from build123d import *

# Parameters (mm, degrees)
PAD_DEPTH         = 10
SKETCH001_W       = 10
SKETCH001_H       = 4
SKETCH001_W_2     = 3
POCKET_DEPTH      = 18.580627
POCKET_DEPTH_BACK = -1.421373
SKETCH002_R       = 1.6
POCKET001_DEPTH   = 6.001
SKETCH003_R       = 3.1
POCKET002_DEPTH   = 3
SKETCH004_W       = 2.736464
SKETCH004_H       = 4
POCKET003_DEPTH   = 5


with BuildPart() as part:
    # Sketch → Pad (new body, symmetric)
    with BuildSketch(Plane.XZ):
        with BuildLine():
            ThreePointArc((-8.737986, 10), (-9.998746, 4.978781), (-8.579627, 0))
            Line((-8.579627, 0), (-8.579627, -6))
            Line((-8.579627, -6), (8.579627, -6))
            Line((8.579627, -6), (8.579627, 0))
            ThreePointArc((8.579627, 0), (9.998746, 4.978781), (8.737986, 10))
            Line((5.843163, 6.5), (8.737986, 10))
            ThreePointArc((3.1, 0), (5.527888, 2.804212), (5.843163, 6.5))
            Line((-3.1, 0), (3.1, 0))
            ThreePointArc((-5.843163, 6.5), (-5.527888, 2.804212), (-3.1, 0))
            Line((-5.843163, 6.5), (-8.737986, 10))
        make_face()
    extrude(amount=PAD_DEPTH, both=True)

    # Sketch001 (on Face5 of Pad) → Pocket (cut, two sides)
    with BuildSketch(Plane(origin=(8.579627, 0, 0), x_dir=(0, 0, 1), z_dir=(1, 0, 0))) as pocket_sk:
        with Locations((5, 0)):
            Rectangle(SKETCH001_W, SKETCH001_H)
        with Locations((-4.5, 0)):
            Rectangle(SKETCH001_W_2, SKETCH001_H)
    extrude(amount=-POCKET_DEPTH, mode=Mode.SUBTRACT)
    extrude(pocket_sk.sketch, amount=-POCKET_DEPTH_BACK, mode=Mode.SUBTRACT)

    # Sketch002 (on Face12 of Pocket) → Pocket001 (cut, through all)
    with BuildSketch(Plane(origin=(0, 0, 0), x_dir=(-1, 0, 0), z_dir=(0, 0, 1))):
        with Locations((0, 6)):
            Circle(SKETCH002_R)
        with Locations((0, -6)):
            Circle(SKETCH002_R)
    extrude(amount=-POCKET001_DEPTH, mode=Mode.SUBTRACT)

    # Sketch003 (on Face30 of Pocket001) → Pocket002 (cut)
    with BuildSketch(Plane(origin=(0, 0, 0), x_dir=(-1, 0, 0), z_dir=(0, 0, 1))):
        with Locations((0, 6)):
            Circle(SKETCH003_R)
        with Locations((0, -6)):
            Circle(SKETCH003_R)
    extrude(amount=-POCKET002_DEPTH, mode=Mode.SUBTRACT)

    # Sketch004 (on Face13 of Pocket002) → Pocket003 (cut)
    with BuildSketch(Plane(origin=(0, 0, 0), x_dir=(-1, 0, 0), z_dir=(0, 0, 1))):
        with Locations((-7.211395, 0)):
            Rectangle(SKETCH004_W, SKETCH004_H)
        with Locations((7.211395, 0)):
            Rectangle(SKETCH004_W, SKETCH004_H)
    extrude(amount=-POCKET003_DEPTH, mode=Mode.SUBTRACT)


solid = part.part
Can you work these out from the model? Positions are in its coordinate system, mm. A direction names the side the tool comes from. Give positions to 0.01 mm unless a question says otherwise; leave off trailing zeros. Order: outer loops, then holes, each group sorted by start corner. A loop starts at its lowest first (then second) coordinate and runs counter-clockwise, first axis right, second up. Notation, with made-up numbers: M 73.5,67 L 86.5,67 A15 ccw 86.5,85 Z; hole C 69,62.5 d11. An arc over 180 degrees is marked long. One line per question, with ' | ' between items.
Item 1: Please list where these lines run through material, in increasing order: L1, parallel to Y at x = 0, z = -5; L2, parallel to Y at x = 0, z = -1.8; L3, parallel to X at y = 6, z = -0.7.
Answer block:
L1: y = -10 to -7.6, -4.4 to -2, 2 to 4.4, 7.6 to 10 | L2: y = -10 to -9.1, -2.9 to 2.9, 9.1 to 10 | L3: x = -8.58 to -3.1, 3.1 to 8.58
Item 2: I'm going to push flat-ended pins straight in: pin 1 Ø1.8 at (y, z) = (-4, -2.5) entering from -X; pin 2 Ø5 at (x, y) = (-1.5, 5.5) entering from +Z (3 decimals); pin 3 Ø2 at (y, z) = (-3, 7) entering from -X; pin 4 Ø5 at (x, z) = (1, 3.5) entering from +Y. Where does each tip first touch, or does it pass through?
Answer block:
pin 1: stops at x = -8.58 | pin 2: stops at z = 0.665 | pin 3: stops at x = -9.96 | pin 4: passes through
Item 3: For faces 1 (the face through (-5.843, 0, -1)), 2 (the face through (-5.548, -6.056, 2.853)), 3 (the face through (0.672, -2.974, -1.479)), 4 (the face through (-7.27, 5.944, 8.226)), 5 (the face through (8.58, 6, -3)), which set-ups out of +Z, -Z, +X, -X, +Y, -Y let a thin tool reach every point of the face, with its end or its side?
Answer block:
face 1: +Z, -Z, -X | face 2: +Y, -Y | face 3: +Z | face 4: +Z, +Y, -Y | face 5: -Z, +X, +Y, -Y
Item 4: Suppose I cut it at C-C, the plane z = -0.5. Write out the boundary of the cut face in (x, y).
Answer block:
outline: M -8.58,-10 L 8.58,-10 L 8.58,-2 L 5.84,-2 L 5.84,2 L 8.58,2 L 8.58,10 L -8.58,10 L -8.58,2 L -5.84,2 L -5.84,-2 L -8.58,-2 Z; hole C 0,-6 d6.2; hole C 0,6 d6.2
Item 5: Suppose I cut it at D-D, the plane z = 7.75. Write out the boundary of the cut face in (x, y), then the cut area to 3 significant figures.
Answer block:
outline: M -9.65,-10 L -6.88,-10 L -6.88,-2 L -9.65,-2 Z; M -9.65,2 L -6.88,2 L -6.88,10 L -9.65,10 Z; M 6.88,-10 L 9.65,-10 L 9.65,-2 L 6.88,-2 Z; M 6.88,2 L 9.65,2 L 9.65,10 L 6.88,10 Z | area: 88.8 mm2
Item 6: Suppose I cut it at A-A, the plane z = -3.75. Write out the boundary of the cut face in (x, y).
Answer block:
outline: M -8.58,-10 L 8.58,-10 L 8.58,-2 L -8.58,-2 Z; M -8.58,2 L 8.58,2 L 8.58,10 L -8.58,10 Z; hole C 0,-6 d3.2; hole C 0,6 d3.2
Item 7: We'd pull the mould along X, two halves only. Please class faces 6 (the face through (10, 6, 5)), 7 (the face through (-8.58, 6, -3)), 8 (the face through (-5.548, 5.944, 2.853)), 9 (the face through (0, -10, -1)): released by +X, released by -X, zero draft, split by the parting line, or undercut.
Answer block:
face 6: released by +X | face 7: released by -X | face 8: undercut | face 9: zero draft
Item 8: Suppose I cut it at B-B, the plane x = 0. Write out the boundary of the cut face in (y, z).
Answer block:
outline: M -10,-6 L -7.6,-6 L -7.6,-3 L -9.1,-3 L -9.1,0 L -10,0 Z; M -4.4,-6 L -2,-6 L -2,-3 L 2,-3 L 2,-6 L 4.4,-6 L 4.4,-3 L 2.9,-3 L 2.9,0 L -2.9,0 L -2.9,-3 L -4.4,-3 Z; M 7.6,-6 L 10,-6 L 10,0 L 9.1,0 L 9.1,-3 L 7.6,-3 Z
